Work out the finished part from the listing and answer in its coordinate system (mm). Face numbers are marked on the shaded views. A direction names the side the tool comes from. Coordinates: 2 decimals unless noted, no trailing zeros. Order: outer loops, then holes, each group sorted by start corner. A loop starts at its lowest first (then second) coordinate and runs counter-clockwise, first axis right, second up. Notation, with made-up numbers: M 72,34.5 L 125,34.5 A34 cw 125,67.5 Z; hole C 57.5,39.5 d8. An arc over 180 degrees is marked long. Write item = value, one per line. Start each with the question number.
Q1. Straight lines are drawn through the part: line 1 along Y through (x, z) = (0, 5.7); line 2 along Y through (x, z) = (-14, 6); line 3 along X through (y, z) = (-15.5, 2). For each, find the intervals that lie inside material, in ascending order.
Q2. Determine the mould class of the marked faces 1, 2, 3 and 4 for opening direction X: released by +X, released by -X, zero draft, split by the parting line, or undercut.
Q3. Each of these flat-tipped pins is pushed along its axis until it touches: P1, Ø1.5, axis at x = 14.5, z = 2, coming from the -Y side; P2, Ø2, axis at x = -0.5, y = -3.5, coming from the -Z side; P3, Ø3, axis at y = 0, z = 6.5, coming from the -X side; P4, Ø1.1, axis at x = 0, y = -14.45, coming from the +Z side. Where does it stop, or does it pass through?
Q4. Find section C-C on x = 7. Give the vertices of the cut face in (y, z).
Q5. Find section A-A on y = 0. Give the vertices of the cut face in (x, z).
Q6. Find section B-B on z = 6.25. Give the number of separate pieces and of enclosed holes in the cut face, and give its area (3 significant figures).
Q7. A tool of negligible diameter and unlimited length cuts with its end or side. For the marked faces 5, 6 and 7, from which of +Z, -Z, +X, -X, +Y, -Y can it reach the whole face along a straight path? Write none if from no direction.
```python
from build123d import *

# Parameters (mm, degrees)
SKETCH1_R           = 19
BOSS_EXTRUDE2_DEPTH = 7
BOSS_EXTRUDE3_DEPTH = 7
CIRPATTERN1_COUNT   = 26
SKETCH1_7_R         = 0.6
CUT_EXTRUDE1_DEPTH  = 4
SKETCH1_8_R         = 0.6
CUT_EXTRUDE2_DEPTH  = 7


with BuildPart() as part:
    # Sketch1 → Boss-Extrude2 (new body)
    with BuildSketch(Plane.XY):
        Circle(SKETCH1_R)
    extrude(amount=BOSS_EXTRUDE2_DEPTH)

    # Sketch1<6> → Boss-Extrude3 (add)
    with BuildSketch(Plane.XY):
        with BuildLine():
            Line((-0.557497486, -21.995033976), (0.242502514, -21.995033976))
            ThreePointArc((0.242502514, -21.995033976), (0.782724682, -20.5339516), (0.883393299, -18.979452476))
            ThreePointArc((0.883393299, -18.979452476), (-0.157029313, -18.999351089), (-1.196980891, -18.962258219))
            ThreePointArc((-1.196980891, -18.962258219), (-1.099506092, -20.525512733), (-0.557497486, -21.995033976))
        make_face()
    boss_extrude3 = extrude(amount=BOSS_EXTRUDE3_DEPTH)

    # CirPattern1: Boss-Extrude3 ×26 about axis
    cirpattern1_axis = Axis((0, 0, 0), (0, 0, 1))
    for i in range(1, CIRPATTERN1_COUNT):
        add(boss_extrude3.rotate(cirpattern1_axis, i * 360 / CIRPATTERN1_COUNT))

    # Sketch1<7> → Cut-Extrude1 (cut)
    with BuildSketch(Plane.XY):
        with BuildLine():
            Line((-2.025, -14.025), (-2.65, -2.286372673))
            ThreePointArc((-2.65, -2.286372673), (0, 3.5), (2.65, -2.286372673))
            Line((2.65, -2.286372673), (2.025, -14.025))
            ThreePointArc((2.025, -14.025), (0, -16.05), (-2.025, -14.025))
        make_face()
        with Locations((0, -14.45)):
            Circle(SKETCH1_7_R, mode=Mode.SUBTRACT)
        with Locations((0, -12.45)):
            Circle(SKETCH1_7_R, mode=Mode.SUBTRACT)
    extrude(amount=CUT_EXTRUDE1_DEPTH, mode=Mode.SUBTRACT)

    # Sketch1<8> → Cut-Extrude2 (cut)
    with BuildSketch(Plane.XY):
        with Locations((0, -14.45)):
            Circle(SKETCH1_8_R)
        with Locations((0, -12.45)):
            Circle(SKETCH1_8_R)
    extrude(amount=CUT_EXTRUDE2_DEPTH, mode=Mode.SUBTRACT)


solid = part.part
```
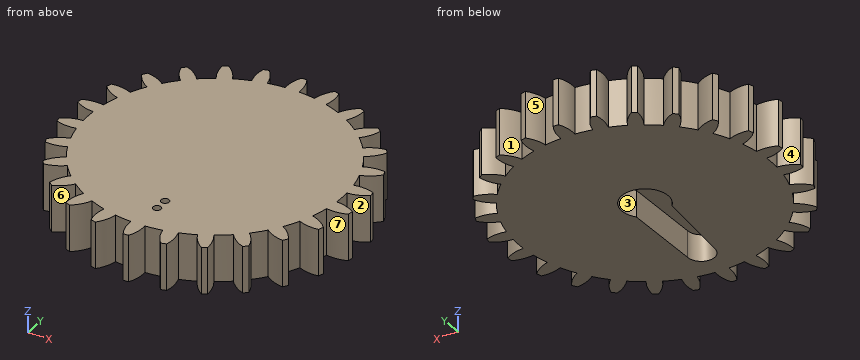
Findings below:
q1.line_1 = -22 to -15.05, -13.85 to -13.05, -11.85 to 22
q1.line_2 = -16.46 to -13.99, -12.85 to 12.85, 14.52 to 16.77
q1.line_3 = -14.83 to -12.56, -10.99 to -1.39, 1.39 to 10.99, 12.11 to 14.52
q2.face_1 = undercut
q2.face_2 = released by +X
q2.face_3 = undercut
q2.face_4 = released by -X
q3.P1 = -16.83
q3.P2 = 4
q3.P3 = -20.82
q3.P4 = through
q4.outline = M -17.66,0 L 17.66,0 L 17.66,7 L -17.66,7 Z
q5.outline = M -19,0 L -3.5,0 L -3.5,4 L 3.5,4 L 3.5,0 L 19,0 L 19,7 L -19,7 Z
q6.separate_pieces = 1
q6.enclosed_holes = 2
q6.area = 1,270 mm^2
q7.face_5 = +Z, -Z, +Y
q7.face_6 = +Z, -Z, -Y
q7.face_7 = +Z, -Z
